Geometry: see drawing. Coordinates: mm, zero at the bounding-box minimum. A direction names the side the tool comes from. Round coordinates to 2 decimals unless told otherwise and drop trailing zeros. Loops run counter-clockwise (first coordinate to the right, second up) from the corner with the lowest first, then second, coordinate; pieces in that order, holes last. Notation, with made-up numbers: (61.25, 0.5) - (117.25, 0.5) arc R15 ccw to (117.25, 8.5) - close; hole circle Ø3 at (76, -16.75). An arc over 180 degrees is marked (long way). Return JSON: item names as keys, results as strings. Group by question number.
1. Section B-B on y = 7.15. Return loops of the section in (x, z).
2. First-contact query: pin 1 Ø1.5 at (x, y) = (10.5, 11) entering from +Z; pin 2 Ø5 at (y, z) = (6, 17) entering from +X; pin 3 Ø0.9 at (x, z) = (7.5, 26.5) entering from -Y. Flat tips, straight axial feed; report the tip coordinate or a pass-through.
3. Draft query along X for the marked faces 4, 5 and 6. Return one class per face: +X half, -X half, draft (parallel to the pull), parting line (faces both ways), or undercut.
4. Set-up query: the marked faces 1, 2 and 3. Return all of +Z, -Z, +X, -X, +Y, -Y with unobstructed straight access to the full face (end or side cutting, diameter ignored); none if empty.
5. Section D-D on y = 4.75. Return loops of the section in (x, z), and give its area (3 significant figures).
6. Material intervals for probe 1 along Y at (x, z) = (7.15, 0.7); probe 2 along Z at (x, y) = (1.75, 4.25); probe 3 along Y at (x, z) = (7.25, 25), sorted ascending.
7. Section A-A on x = 7.15. Return loops of the section in (y, z).
8. Section C-C on z = 23. Return loops of the section in (x, y).
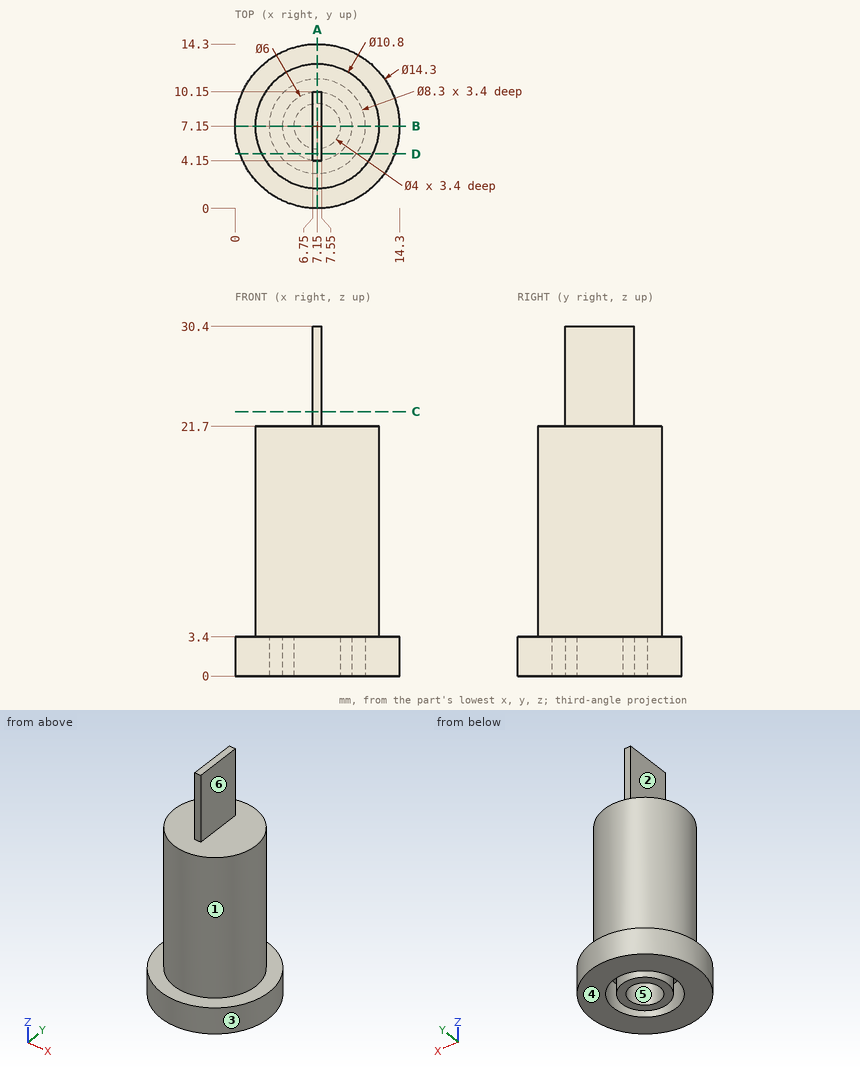
Taken from the geometry:
{
 "1": {"outline": "(0, 0) - (3, 0) - (3, 3.4) - (4.15, 3.4) - (4.15, 0) - (5.15, 0) - (5.15, 3.4) - (9.15, 3.4) - (9.15, 0) - (10.15, 0) - (10.15, 3.4) - (11.3, 3.4) - (11.3, 0) - (14.3, 0) - (14.3, 3.4) - (12.55, 3.4) - (12.55, 21.7) - (7.55, 21.7) - (7.55, 30.4) - (6.75, 30.4) - (6.75, 21.7) - (1.75, 21.7) - (1.75, 3.4) - (0, 3.4) - close"},
 "2": {"pin 1": "z = 21.7", "pin 2": "x = 12.55", "pin 3": "y = 4.15"},
 "3": {"face 4": "draft", "face 5": "undercut", "face 6": "+X half"},
 "4": {"face 1": "+Z", "face 2": "+Z, -X, +Y, -Y", "face 3": "+Z, -Z"},
 "5": {"outline": "(0.41, 0) - (3.76, 0) - (3.76, 3.4) - (5.35, 3.4) - (5.35, 0) - (8.95, 0) - (8.95, 3.4) - (10.54, 3.4) - (10.54, 0) - (13.89, 0) - (13.89, 3.4) - (11.99, 3.4) - (11.99, 21.7) - (7.55, 21.7) - (7.55, 30.4) - (6.75, 30.4) - (6.75, 21.7) - (2.31, 21.7) - (2.31, 3.4) - (0.41, 3.4) - close", "area": "219 mm2"},
 "6": {"probe 1": "0 to 3, 4.15 to 5.15, 9.15 to 10.15, 11.3 to 14.3", "probe 2": "0 to 3.4", "probe 3": "4.15 to 10.15"},
 "7": {"outline": "(0, 0) - (3, 0) - (3, 3.4) - (4.15, 3.4) - (4.15, 0) - (5.15, 0) - (5.15, 3.4) - (9.15, 3.4) - (9.15, 0) - (10.15, 0) - (10.15, 3.4) - (11.3, 3.4) - (11.3, 0) - (14.3, 0) - (14.3, 3.4) - (12.55, 3.4) - (12.55, 21.7) - (10.15, 21.7) - (10.15, 30.4) - (4.15, 30.4) - (4.15, 21.7) - (1.75, 21.7) - (1.75, 3.4) - (0, 3.4) - close"},
 "8": {"outline": "(6.75, 4.15) - (7.55, 4.15) - (7.55, 10.15) - (6.75, 10.15) - close"}
}
